CAD build for the part. Positions are in the model's coordinates, mm. A direction names the side the tool comes from. Round coordinates to 2 decimals unless told otherwise and drop trailing zeros. Order: outer loops, then holes, each group sorted by start corner. A loop starts at its lowest first (then second) coordinate and runs counter-clockwise, first axis right, second up. Notation, with made-up numbers: M 11,-29.75 L 55,-29.75 A27 cw 55,-7.75 Z; hole C -34.5,83 d1. An arc over 180 degrees is marked long. Answer as a JSON object with one key per item and string values.
Autodesk Inventor part; units mm, degrees
ref_plane "YZ Plane" through (0, 0, 0) normal (1, 0, 0) x (0, 1, 0)
ref_plane "XZ Plane" through (0, 0, 0) normal (0, 1, 0) x (-1, 0, 0)
ref_plane "XY Plane" through (0, 0, 0) normal (0, 0, 1) x (1, 0, 0)
sketch "Sketch1" plane through (0, 0, 0) normal (0, 1, 0) x (-1, 0, 0)
  line L0 (17.529, 129.5854) -> (-122.471, 129.5854)
  line L1 (-122.471, 129.5854) -> (-122.471, -30.4146)
  line L2 (-122.471, -30.4146) -> (17.529, -30.4146)
  line L3 (17.529, -30.4146) -> (17.529, 129.5854)
  point P0 (0, 0)
  dimension "d0" = 160
  dimension "d1" = 140
extrude "Extrusion1" add sketch "Sketch1" along normal blind 4
sketch "Sketch2" plane through (0, 4, 0) normal (0, 1, 0) x (1, 0, 0)
  point P0 (0, 0)
sketch "Sketch3" plane through (0, 4, 0) normal (0, 1, 0) x (1, 0, 0)
  line L0 (17.471, -114.5854) -> (87.471, -114.5854)
  line L1 (87.471, -114.5854) -> (87.471, -64.5854)
  line L2 (87.471, -64.5854) -> (17.471, -64.5854)
  line L3 (17.471, -64.5854) -> (17.471, -114.5854)
  line L4 (-7.529, -49.5854) -> (42.471, -49.5854)
  line L5 (42.471, -49.5854) -> (42.471, 20.4146)
  line L6 (42.471, 20.4146) -> (-7.529, 20.4146)
  line L7 (-7.529, 20.4146) -> (-7.529, -49.5854)
  line L8 (62.471, -49.5854) -> (112.471, -49.5854)
  line L9 (112.471, -49.5854) -> (112.471, 20.4146)
  line L10 (112.471, 20.4146) -> (62.471, 20.4146)
  line L11 (62.471, 20.4146) -> (62.471, -49.5854)
  line L12 (-17.529, -129.5854) -> (122.471, -129.5854)
  line L13 (-17.529, 30.4146) -> (-17.529, -129.5854)
  line L14 (122.471, 30.4146) -> (-17.529, 30.4146)
  line L15 (122.471, -129.5854) -> (122.471, 30.4146)
  point P0 (0, 0)
  dimension "d4" = 50
  dimension "d5" = 70
  dimension "d6" = 50
  dimension "d7" = 50
  dimension "d8" = 70
  dimension "d9" = 70
  dimension "d10" = 15
  dimension "d11" = 10
  dimension "d12" = 10
  dimension "d13" = 10
  dimension "d14" = 10
  dimension "d15" = 35
  dimension "d16" = 35
extrude "Extrusion2" add sketch "Sketch3" along normal blind 4 contours L3 L2 L1 L0 | L7 L6 L5 L4 | L11 L10 L9 L8
properties part number "Stage with Boards"
Item 1: Saw through at C-C on x = 54.5. List the corners of the cut face in (y, z).
Worked answers:
{"outline": "M 0,-30.41 L 4,-30.41 L 4,64.59 L 8,64.59 L 8,114.59 L 4,114.59 L 4,129.59 L 0,129.59 Z"}
Item 2: Wall check: line 1 along X through (y, z) = (6.5, -14); line 2 along Z through (x, y) = (40, 7); line 3 along Z through (x, y) = (8, 6.5). Give the ranges that are in metal, low to high. Write a range as [from, to].
Worked answers:
{"line 1": "x = [-7.53, 42.47], [62.47, 112.47]", "line 2": "z = [-20.41, 49.59], [64.59, 114.59]", "line 3": "z = [-20.41, 49.59]"}
Item 3: Saw through at B-B on z = -11.5. List the corners of the cut face in (x, y), and give its area (3 significant figures).
Worked answers:
{"outline": "M -17.53,0 L 122.47,0 L 122.47,4 L 112.47,4 L 112.47,8 L 62.47,8 L 62.47,4 L 42.47,4 L 42.47,8 L -7.53,8 L -7.53,4 L -17.53,4 Z", "area": "960 mm2"}
Item 4: 3-axis set-ups, long thin cutter, end or side, ignore diameter. For faces 1 (the flat face through (17, 6, 49.585)), 2 (the flat face through (17.471, 6, 89)), 3 (the flat face through (18, 6, -20.415)): which of +Z, -Z, +X, -X, +Y, -Y reach the whole face in a straight line?
Worked answers:
{"face 1": "+X, -X, +Y", "face 2": "+Z, -X, +Y", "face 3": "-Z, +X, -X, +Y"}
Item 5: Drop flat-ended pins along their axis: pin 1 Ø3 at (x, y) = (58.5, 6) entering from -Z; pin 2 Ø3 at (y, z) = (6.5, 80.5) entering from +X; pin 3 Ø1.2 at (y, z) = (6.5, 80) entering from -X. Give the stop position or say it passes through.
Worked answers:
{"pin 1": "stops at z = 64.59", "pin 2": "stops at x = 87.47", "pin 3": "stops at x = 17.47"}
Item 6: Two-plate mould, pull along X, no slides. Class faces 4 (the flat face through (-7.529, 6, 14)), 5 (the flat face through (87.471, 6, 90)), 6 (the flat face through (52, 8, 89)), 7 (the flat face through (62.471, 6, 14)): released by +X, released by -X, zero draft, split by the parting line, or undercut.
Worked answers:
{"face 4": "released by -X", "face 5": "released by +X", "face 6": "zero draft", "face 7": "undercut"}
Item 7: Saw through at D-D on z = 80. List the corners of the cut face in (x, y), and give its area (3 significant figures).
Worked answers:
{"outline": "M -17.53,0 L 122.47,0 L 122.47,4 L 87.47,4 L 87.47,8 L 17.47,8 L 17.47,4 L -17.53,4 Z", "area": "840 mm2"}
Item 8: Saw through at A-A on y = 6.5. List the corners of the cut face in (x, z).
Worked answers:
{"outline": "M -7.53,-20.41 L 42.47,-20.41 L 42.47,49.59 L -7.53,49.59 Z; M 17.47,64.59 L 87.47,64.59 L 87.47,114.59 L 17.47,114.59 Z; M 62.47,-20.41 L 112.47,-20.41 L 112.47,49.59 L 62.47,49.59 Z"}
